Autodesk Inventor part; units mm, degrees
ref_plane "YZ Plane" through (0, 0, 0) normal (1, 0, 0) x (0, 1, 0)
ref_plane "XZ Plane" through (0, 0, 0) normal (0, 1, 0) x (-1, 0, 0)
ref_plane "XY Plane" through (0, 0, 0) normal (0, 0, 1) x (1, 0, 0)
sketch "Sketch1" plane through (0, 0, 0) normal (0, 0, 1) x (1, 0, 0)
  line L0 (-3.3676, 3.3676) -> (3.3676, 3.3676)
  line L1 (3.3676, 3.3676) -> (3.3676, -3.3676)
  line L2 (3.3676, -3.3676) -> (-3.3676, -3.3676)
  line L3 (-3.3676, -3.3676) -> (-3.3676, 3.3676)
  line L4 (-3.3676, 3.3676) -> (3.3676, -3.3676) construction
  line L5 (3.3676, 3.3676) -> (-3.3676, -3.3676) construction
  point P0 (0, 0)
  dimension "d0" = 6.7352
extrude "Extrusion1" add sketch "Sketch1" along normal blind 6.35
sketch "Sketch2" plane through (0, 0, 6.35) normal (0, 0, 1) x (1, 0, 0)
  line L0 (3.3676, -3.3676) -> (3.3676, 3.3676)
  line L1 (-3.3676, -3.3676) -> (3.3676, -3.3676)
  line L2 (3.3676, 3.3676) -> (-3.3676, 3.3676)
  line L3 (-3.3676, 3.3676) -> (-3.3676, -3.3676)
  circle A0 centre (0, 0) radius 4.7625
extrude "Extrusion2" add sketch "Sketch2" along normal blind 4.7625
sketch "Sketch3" plane through (0, 0, 11.1125) normal (0, 0, 1) x (1, 0, 0)
  circle A0 centre (0, 0) radius 4.7625
  line L0 (0, 0) -> (0, -38.1) construction
  line L1 (-4.7625, 0) -> (-4.7625, -38.1)
  line L2 (4.7625, -38.1) -> (4.7625, 0)
  arc A1 (4.7625, 0) -> (-4.7625, 0) centre (0, 0) ccw
  arc A2 (-4.7625, -38.1) -> (4.7625, -38.1) centre (0, -38.1) ccw
  circle A3 centre (0, 0) radius 4.7625
  point P0 (0, -19.05)
  dimension "d5" = 38.1
extrude "Extrusion3" add sketch "Sketch3" along normal blind 4.7625
sketch "Sketch4" plane through (0, 0, 15.875) normal (0, 0, 1) x (1, 0, 0)
  circle A0 centre (0, -38.1) radius 4.7625
  line L0 (4.7625, 0) -> (4.7625, -38.1)
  arc A1 (-4.7625, -38.1) -> (4.7625, -38.1) centre (0, -38.1) ccw
  line L1 (-4.7625, -38.1) -> (-4.7625, 0)
  arc A2 (4.7625, 0) -> (-4.7625, 0) centre (0, 0) ccw
  arc A3 (-4.7625, -38.1) -> (4.7625, -38.1) centre (0, -38.1) ccw
extrude "Extrusion4" add sketch "Sketch4" along normal blind 19.05 contours A0
sketch "Sketch5" plane through (-3.3676, -3.3676, 0) normal (-1, 0, 0) x (0, 0, 1)
  point P0 (0, 3.3676)
sketch "Sketch6" plane through (0, 0, 15.875) normal (0, 0, 1) x (1, 0, 0)
  circle A0 centre (0, 0) radius 4.7625
  line L0 (4.7625, 0) -> (4.7625, -38.1)
  arc A1 (-4.7625, -38.1) -> (4.7625, -38.1) centre (0, -38.1) ccw
  arc A2 (4.7625, -38.1) -> (-4.7625, -38.1) centre (0, -38.1) ccw
  arc A3 (4.7625, 0) -> (-4.7625, 0) centre (0, 0) ccw
  line L1 (-4.7625, -38.1) -> (-4.7625, 0)
hole "Hole1" at (0, 0, 15.875) direction (0, 0, -1) diameter 3.4036 end through all counterbore diameter 6.5024 counterbore depth 2.9972
equation "\"d0\" = l_key"
equation "\"d1\" = d_key"
equation "\"d6\" = t"
equation "\"d8\" = 4 * t"
properties part number "Crank" material "ABS Plastic"
Check sheet for the modelled part. Datum: model origin and axes. Units: mm. A direction names the side the tool comes from. Give positions to 0.01 mm unless a question says otherwise; leave off trailing zeros. Write each loop counter-clockwise with the first axis right and the second up, starting at its lowest first coordinate (ties: lowest second). Pieces come first, ordered by that corner, then holes. Notation, with made-up numbers: (57, 9) -> (89, 9) arc R20 ccw to (89, 24) -> close; hole circle Ø6 at (60, 23). An arc over 180 degrees is marked (long way). Use one line per item in the form item = value. Start each with the question number.
1. Mould release check, pull along X, two halves, no side actions. Record for faces 5 (the cylindrical face through (-1.03, 4.65, 9.99)), 6 (the flat face through (1.4, -1.4, 12.878)), 7 (the flat face through (3.368, 0, 3)), 8 (the flat face through (0, 4, 6.35)): pulls with the +X half, pulls with the -X half, needs draft (parallel to the pull), parting line crosses it, or undercut.
2. Section check D-D (y = -36). Record the cut outline in (x, z) (1 decimal), and give its area (3 significant figures).
3. Thickness scan on line 1 along Y through (x, z) = (0, 13.6); line 2 along X through (y, z) = (0, 3.5); line 3 along X through (y, z) = (0, 13.5). Record the ranges inside material, lowest first. Write a range as from..to.
4. Access from +Z, -Z, +X, -X, +Y, -Y to the whole of each face (thin tool, end or side, straight path). Record for faces 1 (the flat face through (-4, 0, 6.35)), 2 (the flat face through (4, 0, 6.35)), 3 (the cylindrical face through (-3.224, 0.423, 14.355)), 4 (the flat face through (0, 3.368, 3)).
5. Go/stop test with flat-tipped pins: P1, Ø5, axis at y = -0.5, z = 3, coming from the -X side; P2, Ø5, axis at x = 0, y = 0, coming from the +Z side; P3, Ø1.1, axis at x = 0, y = -4, coming from the -Z side. Record where each tip stops, or that it passes through.
6. Section check C-C (z = 29). Record the cut outline in (x, y) (1 decimal).
Conclusion:
q1.face_5 = parting line crosses it
q1.face_6 = undercut
q1.face_7 = pulls with the +X half
q1.face_8 = needs draft
q2.outline = (-4.8, 11.1) -> (4.8, 11.1) -> (4.8, 15.9) -> (4.3, 15.9) -> (4.3, 34.9) -> (-4.3, 34.9) -> (-4.3, 15.9) -> (-4.8, 15.9) -> close
q2.area = 208 mm²
q3.line_1 = -42.86..-3.25, 3.25..4.76
q3.line_2 = -3.37..-1.7, 1.7..3.37
q3.line_3 = -4.76..-3.25, 3.25..4.76
q4.face_1 = -Z, -X, +Y, -Y
q4.face_2 = -Z, +X, +Y, -Y
q4.face_3 = +Z
q4.face_4 = -Z, +X, -X, +Y
q5.P1 = -3.37
q5.P2 = 12.88
q5.P3 = 6.35
q6.outline = circle Ø9.5 at (0, -38.1)
